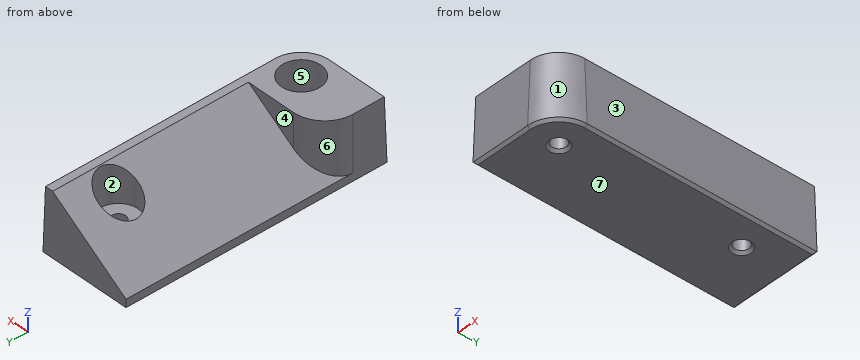
Autodesk Inventor part; units mm, degrees
ref_plane "YZ Plane" through (0, 0, 0) normal (1, 0, 0) x (0, 1, 0)
ref_plane "XZ Plane" through (0, 0, 0) normal (0, 1, 0) x (-1, 0, 0)
ref_plane "XY Plane" through (0, 0, 0) normal (0, 0, 1) x (1, 0, 0)
sketch "Sketch1" plane through (0, 0, 0) normal (0, 0, 1) x (1, 0, 0)
  circle A0 centre (0, 0) radius 12
  line L0 (12, 0) -> (12, 88)
  line L1 (12, 88) -> (-23, 88)
  line L2 (-23, 88) -> (-23, -12)
  line L3 (-23, -12) -> (0, -12)
  dimension "d0" = 24
  dimension "d1" = 100
  dimension "d2" = 35
extrude "Extrusion1" add sketch "Sketch1" along normal blind 25
draft "FaceDraft1" angle 2.5 pull direction (0, 0, 1) faces at (-15.3333, -12, 16.6667) (11.866, -1.7885, 16.6667) (12, 29.3333, 16.6667) fixed edges at (-11.5, -12, 0) (8.4853, -8.4853, 0) (12, 44, 0)
sketch "Sketch2" plane through (0, 0, 0) normal (0, 0, -1) x (-1, 0, 0)
  circle A0 centre (0, 0) radius 2.75
  line L0 (0, 0) -> (0, 102) construction
  circle A1 centre (0, 70) radius 2.75
  dimension "d6" = 5.5
  dimension "d16" = 70
  dimension "d17" = 5.5
extrude "Extrusion2" cut sketch "Sketch2" against normal through all
ref_plane "Work Plane1" through (0, 0, 10) normal (0, 0, -1) x (-1, 0, 0)
sketch "Sketch3" plane through (0, 0, 25) normal (0, 0, 1) x (1, 0, 0)
  circle A0 centre (0, 0) radius 2.75
  circle A1 centre (0, 0) radius 7.5
  circle A2 centre (0, 70) radius 2.75
  circle A3 centre (0, 70) radius 2.75
  circle A4 centre (0, 70) radius 7.5
  dimension "d10" = 15
  dimension "d18" = 15
extrude "Extrusion3" cut sketch "Sketch3" against normal up to surface (15 mm away)
chamfer "Chamfer1" distance 1 angle 45 7 edges at (8.4853, -8.4853, 0) (12, 44, 0) (-11.5, -12, 0) (2.75, 0, 0) (-5.5, 88, 0) (-23, 38, 0) (2.75, 70, 0)
sketch "Sketch4" plane through (-23, 88, 25) normal (0, 1, 0) x (1, 0, 0)
  line L0 (33.9085, 0) -> (0, 0)
  line L1 (0, 24) -> (0, 0)
  line L2 (0, 24) -> (0, 21)
  line L3 (0, 24) -> (0, 0)
  line L4 (34.9564, 24.001) -> (33.9085, 0)
  line L5 (33.9085, 0) -> (30.9085, 0)
  line L6 (23, 0) -> (33.9085, 0)
  line L7 (0, 21) -> (30.9085, 0)
  point P0 (30.9085, 0)
  dimension "d20" = 3
extrude "Extrusion4" cut sketch "Sketch4" against normal blind 75
fillet "Fillet1" radius 12 1 edges at (-23, 13, 14.5)
equation "\"d17\" = d6"
equation "\"d18\" = d10"
properties part number "Holder_3DPrint"
Design review of the part built by this model. Coordinates are the model's own, in mm. Face numbers are marked on the shaded views. A direction names the side the tool comes from. Give positions to 0.01 mm unless a question says otherwise; leave off trailing zeros. Order: outer loops, then holes, each group sorted by start corner. A loop starts at its lowest first (then second) coordinate and runs counter-clockwise, first axis right, second up. Notation, with made-up numbers: (61, 54) - (108, 54) arc R34 ccw to (108, 86) - close; hole circle Ø3 at (83, 33). An arc over 180 degrees is marked (long way). Write item = value, one per line. Start each with the question number.
Q1. We need section C-C on y = 70. State the section outline as (x, z) points, plus the area to 3 significant figures.
Q2. We need section B-B on z = 21.25. State the section outline as (x, y) points.
Q3. Mouldability with a two-part tool opening along Y and no side actions: class the marked faces 1, 2, 3 and 4 as released by +Y, released by -Y, zero draft, split by the parting line, or undercut.
Q4. We need section D-D on x = -12. State the section outline as (y, z) points.
Q5. We need section A-A on y = 25. State the section outline as (x, z) points, plus the area to 3 significant figures.
Q6. Clearance check with flat-ended pins moving along their axes: pin 1 Ø12 at (y, z) = (23.5, 21.5) entering from +X; pin 2 Ø7.5 at (x, y) = (-3.5, 69.5) entering from +Z; pin 3 Ø3 at (y, z) = (50.5, 12.5) entering from -X; pin 4 Ø4.5 at (x, y) = (0, 0) entering from +Z. State where each tip first meets the part, or that it passes through.
Q7. Tool access review of the marked faces 5, 6 and 7: name each direction out of +Z, -Z, +X, -X, +Y, -Y from which nothing blocks a thin tool from reaching the whole face with its end or side.
Q8. To check wall thickness, follow L1, parallel to Y at x = 0, z = 7; L2, parallel to X at y = 59.5, z = 1.5; L3, parallel to X at y = 5.5, z = 12.5. State the ranges of each line that lie inside material, in increasing order. Write a range as from..to.
Working result:
q1.outline = (-23, 1) - (-22, 0) - (-3.75, 0) - (-2.75, 1) - (-2.75, 10) - (-7.5, 10) - (-7.5, 14.53) - (-23, 4) - close; (2.75, 1) - (3.75, 0) - (11, 0) - (11.96, 1) - (10.91, 25) - (7.91, 25) - (7.5, 24.72) - (7.5, 10) - (2.75, 10) - close
q1.area = 335 mm²
q2.outline = (-23, -11.07) - (0, -11.07) arc R11.07 ccw to (11.07, 0) - (11.07, 88) - (2.39, 88) - (2.39, 77.11) arc R7.5 cw to (2.39, 62.89) - (2.39, 13) - (-11, 13) arc R12 ccw to (-23, 1) - close; hole circle Ø15 at (0, 0)
q3.face_1 = released by -Y
q3.face_2 = undercut
q3.face_3 = zero draft
q3.face_4 = released by +Y
q4.outline = (-11.96, 1) - (-11, 0) - (87, 0) - (88, 1) - (88, 11.47) - (12.96, 11.47) - (12.96, 25) - (-10.91, 25) - close
q5.outline = (-23, 1) - (-22, 0) - (11, 0) - (11.96, 1) - (10.91, 25) - (7.91, 25) - (-23, 4) - close
q5.area = 536 mm²
q6.pin_1 = 11.32
q6.pin_2 = 10
q6.pin_3 = -12.7
q6.pin_4 = through
q7.face_5 = +Z
q7.face_6 = +Z, -X, +Y
q7.face_7 = -Z, +X, -X, +Y, -Y
q8.L1 = -11.69..-2.75, 2.75..67.25, 72.75..88
q8.L2 = -23..11.93
q8.L3 = -22.12..-5.1, 5.1..11.45
